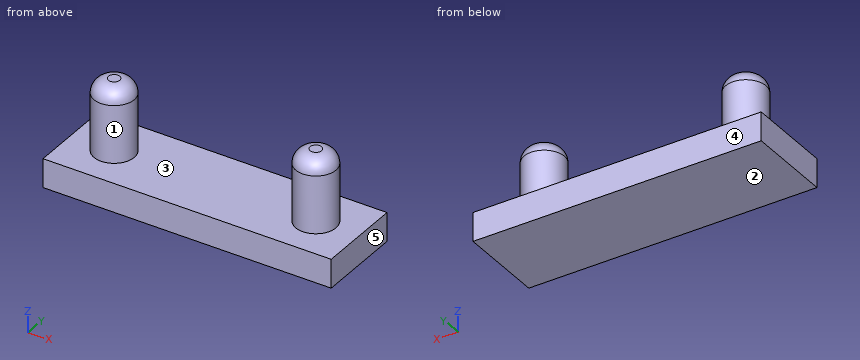
from build123d import *

# Parameters (mm, degrees)
F0_W     = 20
F0_H     = 6
F1_DEPTH = 2
F2_R     = 1.4
F3_DEPTH = 5
F4_R     = 1


with BuildPart() as f1:
    # F0 (on Top) → F1 (new body)
    with BuildSketch(Plane.XY):
        Rectangle(F0_W, F0_H)
    extrude(amount=F1_DEPTH)

    # F2 (on face) → F3 (join)
    with BuildSketch(Plane.XY.offset(2)):
        with Locations((-7, 0)):
            Circle(F2_R)
        with Locations((7, 0)):
            Circle(F2_R)
    extrude(amount=F3_DEPTH)

    # F4
    f4_edges = [f1.edges().sort_by_distance(p)[0] for p in [
        (-8.4, 0, 7),
        (5.6, 0, 7),
    ]]
    fillet(f4_edges, radius=F4_R)


solid = f1.part
Part model, mm, in its own coordinate system. Face numbers are marked on the shaded views. A direction names the side the tool comes from. Give positions to 0.01 mm unless a question says otherwise; leave off trailing zeros. Write each loop counter-clockwise with the first axis right and the second up, starting at its lowest first coordinate (ties: lowest second). Pieces come first, ordered by that corner, then holes.
1) Two-plate mould, pull along X, no slides. Class the marked faces 3, 4 and 5: released by +X, released by -X, zero draft, split by the parting line, or undercut.
Resolved:
face 3: undercut
face 4: zero draft
face 5: released by +X
2) Which spindle directions (+Z, -Z, +X, -X, +Y, -Y) get a long thin tool onto all of the face, cutting with end or side? Do the marked faces 1 and 2. Say none if no direction does.
Resolved:
face 1: +Z
face 2: -Z, +X, -X, +Y, -Y
3) Cut at B-B on x = -2. Write the cut outline in (y, z).
Resolved:
outline: (-3, 0) - (3, 0) - (3, 2) - (-3, 2) - close
4) Probe L1, parallel to Z at x = -6, y = 2.15; L2, parallel to X at y = 0.3, z = 5; L3, parallel to X at y = 1.2, z = 2.75. List the from-to ranges inside material, lowest first.
Resolved:
L1: z = 0 to 2
L2: x = -8.37 to -5.63, 5.63 to 8.37
L3: x = -7.72 to -6.28, 6.28 to 7.72
5) Pin check, flat tip, straight feed: pin 1 (3 mm diameter, centred on y = -1, z = 5, fed in from +X). Stop position of the tip, or through.
Resolved:
pin 1: stops at x = 8.4
6) Cut at A-A on z = 3.5. Write the cut outline in (x, y), then the cut area to 3 significant figures.
Resolved:
outline: circle Ø2.8 at (-7, 0); circle Ø2.8 at (7, 0)
area: 12.3 mm2
